The figure shows three views and two pictorial views of one solid part (mm, origin at its lowest corner). Answer the questions. Give positions to 0.01 mm unless a question says otherwise; leave off trailing zeros. Write each loop counter-clockwise with the first axis right and the second up, starting at its lowest first coordinate (ties: lowest second). Pieces come first, ordered by that corner, then holes. Notation, with made-up numbers: (-30.5, -11.75) -> (-5.5, -11.75) arc R26 cw to (-5.5, 12.25) -> close; hole circle Ø10 at (2, 82.25). An arc over 180 degrees is marked (long way). Answer as CSV lines item,"result". Start each with the question number.
1. The part is cut by section B-B, the plane x = 1.85. Determine the outline of the cut face in (y, z).
2. The part is cut by section D-D, the plane y = 0.3. Determine the outline of the cut face in (x, z).
3. For a pull along X with two mould halves and no side action, classify the marked faces 1, 2 and 3 as pulls with the +X half, pulls with the -X half, needs draft (parallel to the pull), parting line crosses it, or undercut.
4. The part is cut by section A-A, the plane y = 2.5. Determine the outline of the cut face in (x, z).
5. The part is cut by section C-C, the plane z = 1. Determine the outline of the cut face in (x, y), and give its area (3 significant figures).
6. Given pin 1 (1 mm diameter, centred on x = 4.5, z = 3.5, fed in from -Y), flat-ended and moving along its own axis, determine where the tip first touches the part or whether it passes through.
7. Find the intervals of material crossed by line 1 (Y direction, x = 2.5, z = 3.5); line 2 (Y direction, x = 2.5, z = 0.2); line 3 (Z direction, x = 4.5, y = 2.1), in increasing order.
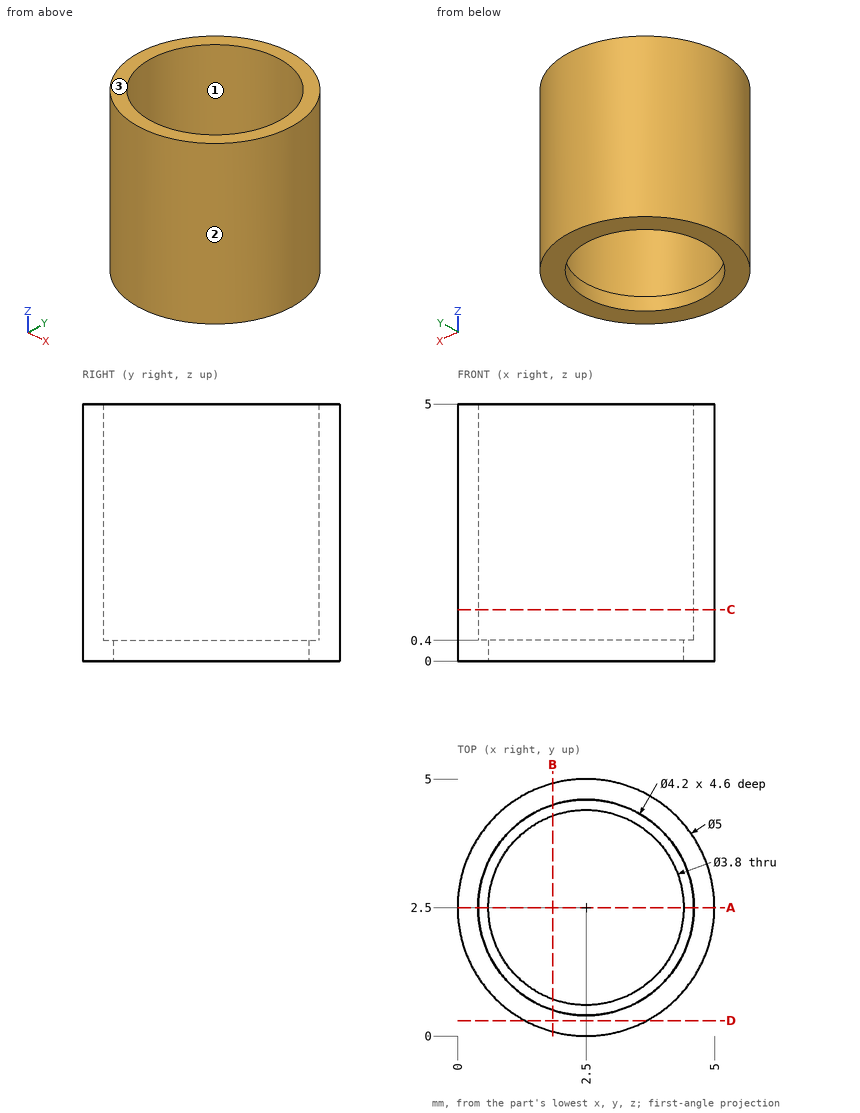
Results found:
1,outline,"(0.09, 0) -> (0.71, 0) -> (0.71, 0.4) -> (0.5, 0.4) -> (0.5, 5) -> (0.09, 5) -> close; (4.29, 0) -> (4.91, 0) -> (4.91, 5) -> (4.5, 5) -> (4.5, 0.4) -> (4.29, 0.4) -> close"
2,outline,"(1.31, 0) -> (3.69, 0) -> (3.69, 5) -> (1.31, 5) -> close"
3,face 1,"undercut"
3,face 2,"parting line crosses it"
3,face 3,"needs draft"
4,outline,"(0, 0) -> (0.6, 0) -> (0.6, 0.4) -> (0.4, 0.4) -> (0.4, 5) -> (0, 5) -> close; (4.4, 0) -> (5, 0) -> (5, 5) -> (4.6, 5) -> (4.6, 0.4) -> (4.4, 0.4) -> close"
5,outline,"circle Ø5 at (2.5, 2.5); hole circle Ø4.2 at (2.5, 2.5)"
5,area,"5.78 mm²"
6,pin 1,"stops at y = 0.5"
7,line 1,"y = 0 to 0.4, 4.6 to 5"
7,line 2,"y = 0 to 0.6, 4.4 to 5"
7,line 3,"z = 0 to 0.4"
